Read the model definition and answer for the solid it produces. Units are mm, in the model's axes. A direction names the side the tool comes from. Give positions to 0.01 mm unless a question says otherwise; leave off trailing zeros. Write each loop counter-clockwise with the first axis right and the second up, starting at its lowest first coordinate (ties: lowest second). Pieces come first, ordered by that corner, then holes. Notation, with made-up numbers: M -22,5 L 4,5 A16 cw 4,15 Z; hole C 40,62.5 d4. An arc over 180 degrees is marked long. Put each result on its own line as item: value.
from build123d import *

# Parameters (mm, degrees)
F0_R     = 12.7
F1_DEPTH = 50.8
F2_W     = 48.538668
F2_H     = 54.82199
F3_DEPTH = 23.8125
F4_W     = 48.538668
F4_H     = 50.8
F5_DEPTH = 76.2
F6_R     = 16.51
F6_R_2   = 12.7
F7_DEPTH = 38.1
F8_W     = 50.8
F8_H     = 6.35
F9_DEPTH = 101.6


with BuildPart() as f1:
    # F0 (on Front) → F1 (new body)
    with BuildSketch(Plane.XZ):
        with BuildLine():
            Line((-25.493682, 35.296235), (-25.493682, -15.503765))
            Line((-25.493682, -15.503765), (12.606318, -15.503765))
            ThreePointArc((12.606318, -15.503765), (38.006318, 9.896235), (12.606318, 35.296235))
            Line((12.606318, 35.296235), (-25.493682, 35.296235))
        make_face()
        with Locations((12.606318, 9.896235)):
            Circle(F0_R, mode=Mode.SUBTRACT)
    extrude(amount=F1_DEPTH)

    # F2 (on Right) → F3 (cut, symmetric)
    with BuildSketch(Plane.YZ):
        with Locations((-25.535175, 9.630844)):
            Rectangle(F2_W, F2_H)
    extrude(amount=F3_DEPTH, both=True, mode=Mode.SUBTRACT)

    # F4 (on face) → F5 (cut)
    with BuildSketch(Plane.YZ.offset(-23.8125)):
        with Locations((-25.535175, 9.896235)):
            Rectangle(F4_W, F4_H)
    extrude(amount=F5_DEPTH, mode=Mode.SUBTRACT)

    # F6 (on face) → F7 (join)
    with BuildSketch(Plane(origin=(-25.493682, 0, 0), x_dir=(0, -1, 0), z_dir=(-1, 0, 0))):
        with Locations((25.4, 9.896235)):
            Circle(F6_R)
        with Locations((25.4, 9.896235)):
            Circle(F6_R_2, mode=Mode.SUBTRACT)
    extrude(amount=F7_DEPTH)

    # F8 (on face) → F9 (cut)
    with BuildSketch(Plane(origin=(-25.493682, 0, 0), x_dir=(0, -1, 0), z_dir=(-1, 0, 0))):
        with Locations((25.4, 32.121235)):
            Rectangle(F8_W, F8_H)
        with Locations((25.4, -12.328765)):
            Rectangle(F8_W, F8_H)
    extrude(amount=-F9_DEPTH, mode=Mode.SUBTRACT)


solid = f1.part
(1) For a pull along Z with two mould halves and no side action, classify faces 1 (the face through (-44.277, -12.712, 10.455)), 2 (the face through (-63.594, -34, 0)), 3 (the face through (-10, -1, -9.154)) as +Z half, -Z half, draft (parallel to the pull), parting line (faces both ways), or undercut.
Result:
face 1: undercut
face 2: draft
face 3: -Z half
(2) Section A-A on z = 1.5 is taken. Determine the outline of the cut face in (x, y).
Result:
outline: M -63.59,-39.62 L -25.49,-39.62 L -25.49,-50.8 L 3.08,-50.8 L 3.08,-49.8 L -23.81,-49.8 L -23.81,-1.27 L 3.08,-1.27 L 3.08,0 L -25.49,0 L -25.49,-11.18 L -63.59,-11.18 L -63.59,-15.87 L -25.49,-15.87 L -25.49,-34.93 L -63.59,-34.93 Z; M 22.13,-50.8 L 36.58,-50.8 L 36.58,-49.8 L 22.13,-49.8 Z; M 22.13,-1.27 L 36.58,-1.27 L 36.58,0 L 22.13,0 Z
(3) Section C-C on x = 23 is taken. Determine the outline of the cut face in (y, z), and give its area (3 significant figures).
Result:
outline: M -50.8,-9.15 L -49.8,-9.15 L -49.8,2.6 L -50.8,2.6 Z; M -50.8,17.19 L -49.8,17.19 L -49.8,28.95 L -50.8,28.95 Z; M -1.27,-9.15 L 0,-9.15 L 0,2.6 L -1.27,2.6 Z; M -1.27,17.19 L 0,17.19 L 0,28.95 L -1.27,28.95 Z
area: 53.2 mm²
(4) Straight lines are drawn through the part: line 1 along Y through (x, z) = (0, -4); line 2 along Z through (x, y) = (-34, -25.4); line 3 along X through (y, z) = (-27, 21.5). For each, find the intervals that lie inside material, in ascending order. Write a range as from..to.
Result:
line 1: y = -50.8..-49.8, -1.27..0
line 2: z = -6.61..-2.8, 22.6..26.41
line 3: x = -25.49..-23.81
(5) Section B-B on y = -25.4 is taken. Determine the outline of the cut face in (x, z).
Result:
outline: M -63.59,-6.61 L -25.49,-6.61 L -25.49,-9.15 L -23.81,-9.15 L -23.81,28.95 L -25.49,28.95 L -25.49,26.41 L -63.59,26.41 L -63.59,22.6 L -25.49,22.6 L -25.49,-2.8 L -63.59,-2.8 Z
(6) Section D-D on z = 14 is taken. Determine the outline of the cut face in (x, y).
Result:
outline: M -63.59,-41.39 L -25.49,-41.39 L -25.49,-50.8 L 0.59,-50.8 L 0.59,-49.8 L -23.81,-49.8 L -23.81,-1.27 L 0.59,-1.27 L 0.59,0 L -25.49,0 L -25.49,-9.41 L -63.59,-9.41 L -63.59,-13.38 L -25.49,-13.38 L -25.49,-37.42 L -63.59,-37.42 Z; M 24.63,-50.8 L 37.67,-50.8 L 37.67,-49.8 L 24.63,-49.8 Z; M 24.63,-1.27 L 37.67,-1.27 L 37.67,0 L 24.63,0 Z
(7) Given pin 1 Ø5 at (y, z) = (-15.5, 5) entering from +X; pin 2 Ø7.5 at (y, z) = (-22, 7.5) entering from -X; pin 3 Ø20.5 at (x, z) = (12.61, 9.9) entering from -Y, each flat-ended and moving along its own axis, determine where each tip first touches the part or whether it passes through.
Result:
pin 1: stops at x = -23.81
pin 2: stops at x = -25.49
pin 3: passes through
(8) Which of the six approach directions +Z, -Z, +X, -X, +Y, -Y give full straight-line access (tool end or side, diameter ignored) to faces 4 (the face through (10.953, -50.295, 22.488)), 5 (the face through (1, -49.805, 1)), 6 (the face through (-25.494, -8, 10))?
Result:
face 4: +Y, -Y
face 5: +Z, -Z, +X
face 6: -X
